Verification items for the finished model (mm, model axes). Face numbers are marked on the shaded views. A direction names the side the tool comes from. Give positions to 0.01 mm unless a question says otherwise; leave off trailing zeros. Write each loop counter-clockwise with the first axis right and the second up, starting at its lowest first coordinate (ties: lowest second). Pieces come first, ordered by that corner, then holes. Notation, with made-up numbers: (-31, 24) -> (26, 24) arc R23 cw to (26, 43) -> close; hole circle Ø10 at (23.25, 49). An arc over 180 degrees is marked (long way). Answer as CSV lines item,"result".
```python
from build123d import *

# Parameters (mm, degrees)
SKETCH1_W               = 33
SKETCH1_H               = 27
BOSS_EXTRUDE1_DEPTH     = 46
SKETCH2_W               = 16.5
SKETCH2_H               = 41
CUT_EXTRUDE1_DEPTH      = 59.200085911
FILLET1_RADIUS          = 16.5
FILLET1_LENGTH          = 10.5
SKETCH3_W               = 13
SKETCH3_H               = 23
CUT_EXTRUDE2_DEPTH      = 9
CUT_EXTRUDE3_DEPTH      = 56.12259065
CUT_EXTRUDE3_DEPTH_BACK = 56.12259065
SKETCH4_R               = 6.5
SKETCH5_R               = 1
CUT_EXTRUDE4_DEPTH      = 8
BOSS_EXTRUDE2_START     = 16.5
BOSS_EXTRUDE2_DEPTH     = 16.5
FILLET2_R               = 4
CUT_EXTRUDE5_DEPTH      = 4
SKETCH8_R               = 1.3
CUT_EXTRUDE6_DEPTH      = 1.75
SKETCH9_R               = 2.35
CUT_EXTRUDE7_DEPTH      = 1
SKETCH10_R              = 0.75
CUT_EXTRUDE8_DEPTH      = 1.75


with BuildPart() as part:
    # Sketch1 → Boss-Extrude1 (new body)
    with BuildSketch(Plane(origin=(0, 0, 0), x_dir=(1, 0, 0), z_dir=(0, 1, 0))):
        Rectangle(SKETCH1_W, SKETCH1_H)
    extrude(amount=BOSS_EXTRUDE1_DEPTH)

    # Sketch2 → Cut-Extrude1 (cut, through all)
    with BuildSketch(Plane(origin=(16.5, 0, 0), x_dir=(0, 0, -1), z_dir=(1, 0, 0))):
        with Locations((-5.25, 25.5)):
            Rectangle(SKETCH2_W, SKETCH2_H)
    extrude(amount=-CUT_EXTRUDE1_DEPTH, mode=Mode.SUBTRACT)

    # Fillet1: full round fillet: the end face becomes a half cylinder, R = half its width
    fillet1_face = Plane((0, 46, -8.25), x_dir=(0, 0, 1), z_dir=(0, 1, 0))  # on the end face: x along it, z out of the body
    fillet1_slab = fillet1_face.offset(-FILLET1_RADIUS / 2) * Box(FILLET1_LENGTH, 2 * FILLET1_RADIUS, FILLET1_RADIUS, mode=Mode.PRIVATE)  # the body's end, R deep
    fillet1_round = Plane((0, 29.5, -8.25), x_dir=(0, 1, 0), z_dir=(0, 0, 1)) * Cylinder(FILLET1_RADIUS, FILLET1_LENGTH, mode=Mode.PRIVATE)  # its axis R under the face
    add(fillet1_slab - fillet1_round, mode=Mode.SUBTRACT)

    # Sketch3 → Cut-Extrude2 (cut)
    with BuildSketch(Plane.XY.offset(-3)):
        with Locations((0, 23)):
            Rectangle(SKETCH3_W, SKETCH3_H)
    extrude(amount=-CUT_EXTRUDE2_DEPTH, mode=Mode.SUBTRACT)

    # Sketch4 → Cut-Extrude3 (cut, two sides: drawn at the far end of the back side and taken through both)
    with BuildSketch(Plane.XY.offset(-12).offset(-CUT_EXTRUDE3_DEPTH_BACK)):
        with Locations((0, 28)):
            Circle(SKETCH4_R)
    extrude(amount=CUT_EXTRUDE3_DEPTH + CUT_EXTRUDE3_DEPTH_BACK, mode=Mode.SUBTRACT)

    # Sketch5 → Cut-Extrude4 (cut)
    with BuildSketch(Plane.XY.offset(-3)):
        with Locations((0, 36.8)):
            Circle(SKETCH5_R)
        with Locations((0, 9.2)):
            Circle(SKETCH5_R)
    extrude(amount=-CUT_EXTRUDE4_DEPTH, mode=Mode.SUBTRACT)

    # Sketch6 → Boss-Extrude2 (add)
    with BuildSketch(Plane.XY.offset(-3).offset(BOSS_EXTRUDE2_START)):
        with BuildLine():
            Line((13.5, 5), (16.5, 5))
            Line((16.5, 5), (16.5, 29.5))
            ThreePointArc((16.5, 29.5), (0, 46), (-16.5, 29.5))
            Line((-16.5, 29.5), (-16.5, 5))
            Line((-16.5, 5), (-13.5, 5))
            Line((-13.5, 5), (-13.5, 8))
            Line((-13.5, 8), (-13.5, 29.5))
            ThreePointArc((-13.5, 29.5), (0, 43), (13.5, 29.5))
            Line((13.5, 29.5), (13.5, 8))
            Line((13.5, 8), (13.5, 5))
        make_face()
    extrude(amount=-BOSS_EXTRUDE2_DEPTH)

    # Fillet2
    # the kernel refuses this fillet: 4 mm, written as the material it takes off along each edge
    with BuildSketch(Plane(origin=(16.5, -10, 13.5), x_dir=(-1, 0, 0), z_dir=(0, 1, 0)), Plane(origin=(-16.5, 29.5, 13.5), x_dir=(1, 0, 0), z_dir=(0, -1, 0)), Plane(origin=(-16.5, -10, -13.5), x_dir=(1, 0, 0), z_dir=(0, 1, 0))) as fillet2_piece_1:
        with BuildLine():
            CenterArc((FILLET2_R, -FILLET2_R), FILLET2_R, 90, 90)
            Line((0, -FILLET2_R), (0, 0))
            Line((0, 0), (FILLET2_R, 0))
        make_face()
    extrude(amount=39.5, mode=Mode.SUBTRACT)
    with BuildSketch(Plane(origin=(16.5, -10, -13.5), x_dir=(-1, 0, 0), z_dir=(0, 1, 0))) as fillet2_piece_2:
        with BuildLine():
            CenterArc((FILLET2_R, FILLET2_R), FILLET2_R, 180, 90)
            Line((0, FILLET2_R), (0, 0))
            Line((0, 0), (FILLET2_R, 0))
        make_face()
    extrude(amount=39.5, mode=Mode.SUBTRACT)
    with BuildSketch(Plane(origin=(0, 29.5, -13.5), x_dir=(-1, 0, 0), z_dir=(0, -1, 0))) as fillet2_piece_3:
        with BuildLine():
            CenterArc((16.5 - FILLET2_R, -FILLET2_R), FILLET2_R, 0, 90)
            Line((16.5, -FILLET2_R), (16.5, 0))
            Line((16.5, 0), (16.5 - FILLET2_R, 0))
        make_face()
    revolve(axis=Axis((0, 29.5, -13.5), (0, 0, -1)), revolution_arc=180, mode=Mode.SUBTRACT)
    with BuildSketch(Plane(origin=(0, 29.5, 13.5), x_dir=(1, 0, 0), z_dir=(0, -1, 0))) as fillet2_piece_4:
        with BuildLine():
            CenterArc((16.5 - FILLET2_R, -FILLET2_R), FILLET2_R, 360, 90)
            Line((16.5, -FILLET2_R), (16.5, 0))
            Line((16.5, 0), (16.5 - FILLET2_R, 0))
        make_face()
    revolve(axis=Axis((0, 29.5, 13.5), (0, 0, 1)), revolution_arc=180, mode=Mode.SUBTRACT)

    # Sketch7 → Cut-Extrude5 (cut)
    with BuildSketch(Plane.XZ):
        with BuildLine():
            Line((-14.09375, 1.747487035), (-0.133928571, 2.49641005))
            ThreePointArc((-0.133928571, 2.49641005), (0, 2.5), (0.133928571, 2.49641005))
            Line((0.133928571, 2.49641005), (14.09375, 1.747487035))
            ThreePointArc((14.09375, 1.747487035), (15.75, 0), (14.09375, -1.747487035))
            Line((14.09375, -1.747487035), (0.133928571, -2.49641005))
            ThreePointArc((0.133928571, -2.49641005), (0, -2.5), (-0.133928571, -2.49641005))
            Line((-0.133928571, -2.49641005), (-14.09375, -1.747487035))
            ThreePointArc((-14.09375, -1.747487035), (-15.75, 0), (-14.09375, 1.747487035))
        make_face()
    extrude(amount=-CUT_EXTRUDE5_DEPTH, mode=Mode.SUBTRACT)

    # Sketch8 → Cut-Extrude6 (cut)
    with BuildSketch(Plane.XZ.offset(-4)):
        with Locations(Location((0, 0, 0), (0, 0, 270))):
            Circle(SKETCH8_R)
    extrude(amount=-CUT_EXTRUDE6_DEPTH, mode=Mode.SUBTRACT)

    # Sketch9 → Cut-Extrude7 (cut)
    with BuildSketch(Plane(origin=(0, 5, 0), x_dir=(1, 0, 0), z_dir=(0, 1, 0))):
        with Locations(Location((0, 0, 0), (0, 0, 270))):
            Circle(SKETCH9_R)
    extrude(amount=-CUT_EXTRUDE7_DEPTH, mode=Mode.SUBTRACT)

    # Sketch10 → Cut-Extrude8 (cut)
    with BuildSketch(Plane.XZ.offset(-4)):
        with Locations(Location((8, 0, 0), (0, 0, 270))):
            Circle(SKETCH10_R)
        with Locations(Location((-8, 0, 0), (0, 0, 270))):
            Circle(SKETCH10_R)
    extrude(amount=-CUT_EXTRUDE8_DEPTH, mode=Mode.SUBTRACT)


solid = part.part
```
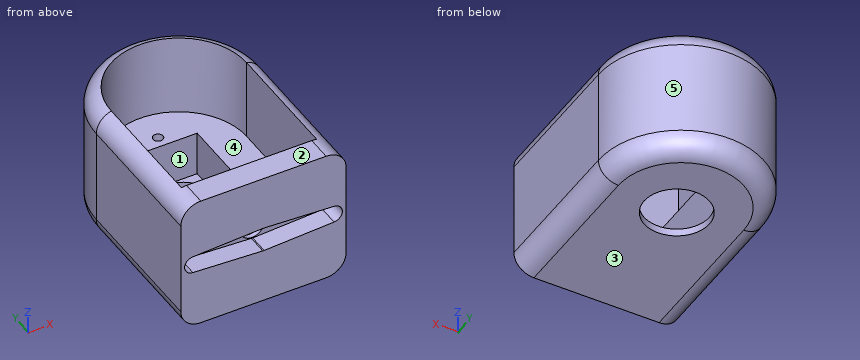
1) Section check B-B (y = 20). Record the boundary of the cut face in (x, z).
Reported:
outline,"(-16.5, -9.5) arc R4 ccw to (-12.5, -13.5) -> (12.5, -13.5) arc R4 ccw to (16.5, -9.5) -> (16.5, 9.5) arc R4 ccw to (13.5, 13.37) -> (13.5, -3) -> (6.5, -3) -> (6.5, -12) -> (-6.5, -12) -> (-6.5, -3) -> (-13.5, -3) -> (-13.5, 13.37) arc R4 ccw to (-16.5, 9.5) -> close"
2) Section check C-C (z = 6.25). Record the boundary of the cut face in (x, y).
Reported:
outline,"(-16.5, 0) -> (16.5, 0) -> (16.5, 29.5) arc R16.5 ccw to (-16.5, 29.5) -> close; hole (-13.5, 5) -> (13.5, 5) -> (13.5, 29.5) arc R13.5 ccw to (-13.5, 29.5) -> close"
3) Section check A-A (z = 0). Record the boundary of the cut face in (x, y), and give its area (3 significant figures).
Reported:
outline,"(-16.5, 0) -> (-15.75, 0) -> (-15.75, 4) -> (-8.75, 4) -> (-8.75, 5) -> (-13.5, 5) -> (-13.5, 29.5) arc R13.5 cw to (13.5, 29.5) -> (13.5, 5) -> (8.75, 5) -> (8.75, 4) -> (15.75, 4) -> (15.75, 0) -> (16.5, 0) -> (16.5, 29.5) arc R16.5 ccw to (-16.5, 29.5) -> close; (-7.25, 4) -> (-2.35, 4) -> (-2.35, 5) -> (-7.25, 5) -> close; (2.35, 4) -> (7.25, 4) -> (7.25, 5) -> (2.35, 5) -> close"
area,"320 mm²"
4) Scan lines: line 1 along Y through (x, z) = (0, -5.25); line 2 along X through (y, z) = (4.35, 0); line 3 along X through (y, z) = (10, 9.75). Record each from-to range of solid material in increasing order.
Reported:
line 1,"0 to 8.2, 10.2 to 11.5, 34.5 to 35.8, 37.8 to 46"
line 2,"-16.5 to -8.75, -7.25 to -2.35, 2.35 to 7.25, 8.75 to 16.5"
line 3,"-16.49 to -13.5, 13.5 to 16.49"
5) Tool access check on the marked faces 1 and 2. Record the directions out of +Z, -Z, +X, -X, +Y, -Y that give a thin tool (end or side, any length) a straight path to the whole face; none if there is none.
Reported:
face 1,"+Z"
face 2,"+Z, +X, -X, +Y, -Y"
6) Depth check by flat-ended pin: pin 1 (0.6 mm diameter, centred on x = 0, y = 36.5, fed in from +Z); pin 2 (5.5 mm diameter, centred on x = 0.5, z = -1, fed in from -Y); pin 3 (17 mm diameter, centred on x = 0, y = 28, fed in from +Z); pin 4 (6.5 mm diameter, centred on x = -1.5, y = 23.5, fed in from +Z). Enter the tip coordinate at first touch or a pass-through.
Reported:
pin 1,"z = -11"
pin 2,"y = 0"
pin 3,"z = -3"
pin 4,"z = -12"
7) Draft check along Y on the marked faces 3, 4 and 5. Enter one of: +Y half, -Y half, draft (parallel to the pull), parting line (faces both ways), or undercut.
Reported:
face 3,"draft"
face 4,"undercut"
face 5,"+Y half"
8) Section check D-D (y = 6.5). Record the boundary of the cut face in (x, z), and give its area (3 significant figures).
Reported:
outline,"(-16.5, -9.5) arc R4 ccw to (-12.5, -13.5) -> (12.5, -13.5) arc R4 ccw to (16.5, -9.5) -> (16.5, 9.5) arc R4 ccw to (13.5, 13.37) -> (13.5, -3) -> (-13.5, -3) -> (-13.5, 13.37) arc R4 ccw to (-16.5, 9.5) -> close"
area,"432 mm²"
